Check sheet for the modelled part. Datum: model origin and axes. Units: mm. Face numbers are marked on the shaded views. A direction names the side the tool comes from. Give positions to 0.01 mm unless a question says otherwise; leave off trailing zeros. Write each loop counter-clockwise with the first axis right and the second up, starting at its lowest first coordinate (ties: lowest second). Pieces come first, ordered by that corner, then holes. Notation, with made-up numbers: (34, 51) -> (46, 51) arc R25 ccw to (46, 84) -> close; hole circle Ø7 at (77.5, 17.25). An arc over 180 degrees is marked (long way). Return JSON: item names as keys, results as strings.
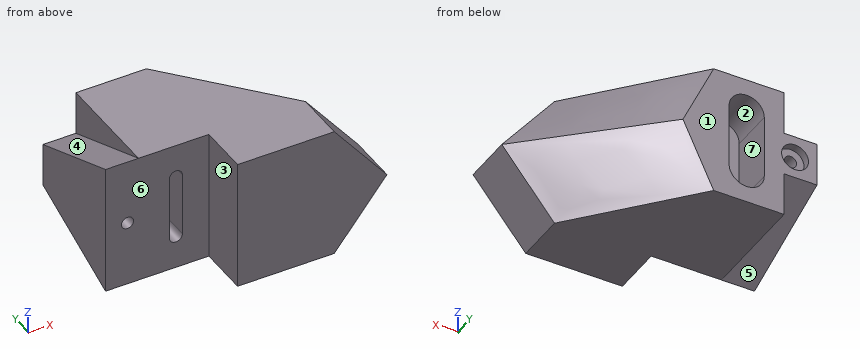
from build123d import *

# Parameters (mm, degrees)
BOSS_EXTRUDE2_DEPTH                     = 23
SKETCH17_W                              = 47
SKETCH17_H                              = 23
CUT_EXTRUDE5_DEPTH                      = 61.0000001
CUT_EXTRUDE6_DEPTH                      = 15
CUT_EXTRUDE7_DEPTH                      = 20
CUT_EXTRUDE8_DEPTH                      = 74.0000001
CBORE_FOR_M5_HEX_HEAD_BOLT2_D           = 5.5
CBORE_FOR_M5_HEX_HEAD_BOLT2_CBORE_D     = 12.24
CBORE_FOR_M5_HEX_HEAD_BOLT2_CBORE_DEPTH = 3.58


with BuildPart() as part:
    # Sketch15 → Loft2 section 0
    with BuildSketch(Plane(origin=(0, 50, 0), x_dir=(1, 0, 0), z_dir=(0, 1, 0))):
        Polygon((0, 30), (0, -30), (47, -30), (61, 0), (47, 30), align=None)
    # Sketch1 → Loft2 section 1
    with BuildSketch(Plane(origin=(0, 0, 0), x_dir=(1, 0, 0), z_dir=(0, 1, 0))):
        Polygon((0, -30), (0, 30), (91, 30), (115, 0), (91, -30), align=None)
    loft()

    # Sketch16 → Boss-Extrude2 (add)
    with BuildSketch(Plane.XZ):
        Polygon((91, 30), (0, 30), (0, -30), (91, -30), (115, 0), align=None)
    extrude(amount=BOSS_EXTRUDE2_DEPTH)

    # Sketch17 → Cut-Extrude5 (cut, through all)
    with BuildSketch(Plane.XY.offset(30)):
        with Locations((23.5, -11.5)):
            Rectangle(SKETCH17_W, SKETCH17_H)
    extrude(amount=-CUT_EXTRUDE5_DEPTH, mode=Mode.SUBTRACT)

    # Sketch19 → Cut-Extrude6 (cut)
    with BuildSketch(Plane.ZY):
        Polygon((10, 50), (30, 50), (30, 0), align=None)
        Polygon((-10, 50), (-30, 50), (-30, 0), align=None)
    extrude(amount=-CUT_EXTRUDE6_DEPTH, mode=Mode.SUBTRACT)

    # Sketch20 → Cut-Extrude7 (cut)
    with BuildSketch(Plane(origin=(0, 50, 0), x_dir=(1, 0, 0), z_dir=(0, 1, 0))):
        with BuildLine():
            Line((40, 14.5), (40, -14.5))
            ThreePointArc((40, -14.5), (32, -22.5), (24, -14.5))
            Line((24, -14.5), (24, 14.5))
            ThreePointArc((24, 14.5), (32, 22.5), (40, 14.5))
        make_face()
        with BuildLine():
            Line((35, 14.5), (35, -14.5))
            ThreePointArc((35, -14.5), (32, -17.5), (29, -14.5))
            Line((29, -14.5), (29, 14.5))
            ThreePointArc((29, 14.5), (32, 17.5), (35, 14.5))
        make_face(mode=Mode.SUBTRACT)
    extrude(amount=-CUT_EXTRUDE7_DEPTH, mode=Mode.SUBTRACT)

    # Sketch20_2 → Cut-Extrude8 (cut, through all)
    with BuildSketch(Plane(origin=(0, 50, 0), x_dir=(1, 0, 0), z_dir=(0, 1, 0))):
        with BuildLine():
            Line((29, 14.5), (29, -14.5))
            ThreePointArc((29, -14.5), (32, -17.5), (35, -14.5))
            Line((35, -14.5), (35, 14.5))
            ThreePointArc((35, 14.5), (32, 17.5), (29, 14.5))
        make_face()
    extrude(amount=-CUT_EXTRUDE8_DEPTH, mode=Mode.SUBTRACT)

    # CBORE for M5 Hex Head Bolt2 (through all)
    with Locations(Plane(origin=(0, 50, 0), x_dir=(1, 0, 0), z_dir=(0, 1, 0))):
        with Locations((10, 0)):
            CounterBoreHole(CBORE_FOR_M5_HEX_HEAD_BOLT2_D / 2, CBORE_FOR_M5_HEX_HEAD_BOLT2_CBORE_D / 2, CBORE_FOR_M5_HEX_HEAD_BOLT2_CBORE_DEPTH)


solid = part.part
(1) Depth check by flat-ended pin: pin 1 Ø16 at (y, z) = (43.5, -2) entering from -X; pin 2 Ø18.5 at (y, z) = (-13, 12.5) entering from -X; pin 3 Ø23 at (y, z) = (17.5, 4.5) entering from +X; pin 4 Ø3 at (y, z) = (21.5, 6.5) entering from +X. Enter the tip coordinate at first touch or a pass-through.
Reply:
{"pin 1": "x = 0", "pin 2": "x = 47", "pin 3": "x = 107.53", "pin 4": "x = 89.36"}
(2) Cross-section at A-A on x = 10. Enter the section's corners in (y, z).
Reply:
{"outline": "(0, -30) -> (50, -10) -> (50, -6.12) -> (46.42, -6.12) -> (46.42, -2.75) -> (0, -2.75) -> close; (0, 2.75) -> (46.42, 2.75) -> (46.42, 6.12) -> (50, 6.12) -> (50, 10) -> (0, 30) -> close"}
(3) Thickness scan on L1, parallel to Y at x = 24, z = 17.5; L2, parallel to Y at x = 38.5, z = -17.5; L3, parallel to Z at x = 11.5, y = 35. Record the ranges inside material, lowest first.
Reply:
{"L1": "0 to 50", "L2": "0 to 30", "L3": "-16 to -2.3, 2.3 to 16"}
(4) Cross-section at B-B on y = 12. State how many separate pieces and enclosed holes the cut face has, then the cut area to 3 significant figures.
Reply:
{"separate pieces": "1", "enclosed holes": "2", "area": "5,100 mm^2"}
(5) Set-up check for the marked faces 4, 5, 6 and 7: record each of +Z, -Z, +X, -X, +Y, -Y from which the full face is reachable in a straight line by a thin tool's end or side.
Reply:
{"face 4": "+Z, -X, +Y", "face 5": "-Z, -X, +Y", "face 6": "+Z, -Z, -X, -Y", "face 7": "+Y"}
(6) Cross-section at C-C on x = 45.5. Enter the section's corners in (y, z).
Reply:
{"outline": "(0, -30) -> (50, -30) -> (50, 30) -> (0, 30) -> close"}
(7) Release check for a two-part mould opening along X. For the marked faces 1, 2 and 3 record: pulls with the +X half, pulls with the -X half, needs draft (parallel to the pull), parting line crosses it, or undercut.
Reply:
{"face 1": "needs draft", "face 2": "undercut", "face 3": "pulls with the -X half"}
